Geometry check sheet. Reference: drawing and pictorial views, mm from the part's lowest x, y, z. A direction names the side the tool comes from. Coordinates: 2 decimals unless noted, no trailing zeros. Write each loop counter-clockwise with the first axis right and the second up, starting at its lowest first coordinate (ties: lowest second). Pieces come first, ordered by that corner, then holes. Notation, with made-up numbers: (19, -8) -> (69, -8) arc R20 ccw to (69, 25) -> close; hole circle Ø11 at (-17, 60.25). An arc over 180 degrees is marked (long way). Answer in a Markdown table with one row per item.
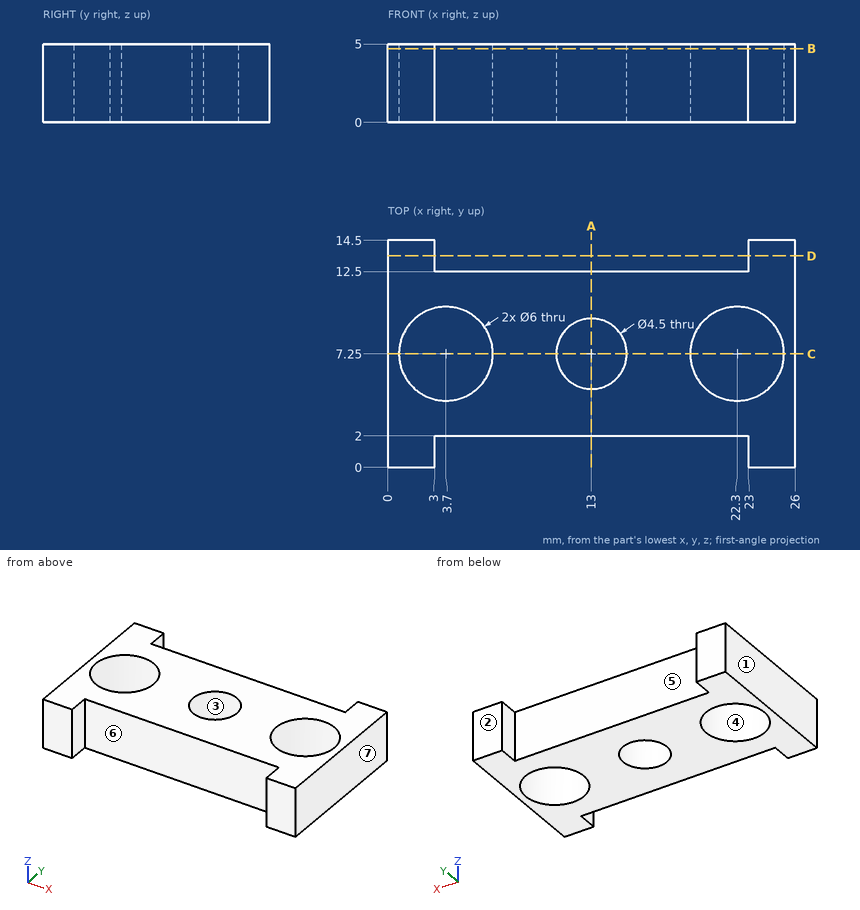
1. Mould release check, pull along X, two halves, no side actions. Record for the marked faces 1, 2, 3 and 4: released by +X, released by -X, zero draft, split by the parting line, or undercut.
Geometry says:
| item | result |
|---|---|
| face 1 | released by -X |
| face 2 | zero draft |
| face 3 | undercut |
| face 4 | undercut |
2. Section check B-B, the plane z = 4.7. Record the boundary of the cut face in (x, y), plus the area to 3 significant figures.
Geometry says:
| item | result |
|---|---|
| outline | (0, 0) -> (3, 0) -> (3, 2) -> (23, 2) -> (23, 0) -> (26, 0) -> (26, 14.5) -> (23, 14.5) -> (23, 12.5) -> (3, 12.5) -> (3, 14.5) -> (0, 14.5) -> close; hole circle Ø6 at (3.7, 7.25); hole circle Ø4.5 at (13, 7.25); hole circle Ø6 at (22.3, 7.25) |
| area | 225 mm^2 |
3. Section check C-C, the plane y = 7.25. Record the boundary of the cut face in (x, z).
Geometry says:
| item | result |
|---|---|
| outline | (0, 0) -> (0.7, 0) -> (0.7, 5) -> (0, 5) -> close; (6.7, 0) -> (10.75, 0) -> (10.75, 5) -> (6.7, 5) -> close; (15.25, 0) -> (19.3, 0) -> (19.3, 5) -> (15.25, 5) -> close; (25.3, 0) -> (26, 0) -> (26, 5) -> (25.3, 5) -> close |
4. Thickness scan on line 1 (Y direction, x = 22.3, z = 3.3); line 2 (Y direction, x = 13, z = 4.7); line 3 (X direction, y = 7.75, z = 1.9). Record the ranges inside material, lowest first. Write a range as from..to.
Geometry says:
| item | result |
|---|---|
| line 1 | 2..4.25, 10.25..12.5 |
| line 2 | 2..5, 9.5..12.5 |
| line 3 | 0..0.74, 6.66..10.81, 15.19..19.34, 25.26..26 |
5. Depth check by flat-ended pin: P1, Ø4, axis at x = 4.5, y = 11, coming from the -Z side; P2, Ø2.5, axis at x = 9, z = 1.5, coming from the +Y side; P3, Ø1.5, axis at x = 10, z = 2, coming from the -Y side. Enter the tip coordinate at first touch or a pass-through.
Geometry says:
| item | result |
|---|---|
| P1 | z = 0 |
| P2 | y = 12.5 |
| P3 | y = 2 |
6. Tool access check on the marked faces 5, 6 and 7. Record the directions out of +Z, -Z, +X, -X, +Y, -Y that give a thin tool (end or side, any length) a straight path to the whole face; none if there is none.
Geometry says:
| item | result |
|---|---|
| face 5 | +Z, -Z, +Y |
| face 6 | +Z, -Z, -Y |
| face 7 | +Z, -Z, +X, +Y, -Y |
7. Section check D-D, the plane y = 13.5. Record the boundary of the cut face in (x, z), plus the area to 3 significant figures.
Geometry says:
| item | result |
|---|---|
| outline | (0, 0) -> (3, 0) -> (3, 5) -> (0, 5) -> close; (23, 0) -> (26, 0) -> (26, 5) -> (23, 5) -> close |
| area | 30.0 mm^2 |
8. Section check A-A, the plane x = 13. Record the boundary of the cut face in (y, z), plus the area to 3 significant figures.
Geometry says:
| item | result |
|---|---|
| outline | (2, 0) -> (5, 0) -> (5, 5) -> (2, 5) -> close; (9.5, 0) -> (12.5, 0) -> (12.5, 5) -> (9.5, 5) -> close |
| area | 30.0 mm^2 |
